Source: CAD feature listing. Evaluate the final solid. Frame: model axes, mm. Face numbers are marked on the shaded views. A direction names the side the tool comes from. Round coordinates to 2 decimals unless told otherwise and drop trailing zeros. Order: outer loops, then holes, each group sorted by start corner. A loop starts at its lowest first (then second) coordinate and runs counter-clockwise, first axis right, second up. Notation, with made-up numbers: (-21, 69) - (19, 69) arc R18 cw to (19, 75) - close; hole circle Ø9 at (-34, 44.5). An arc over 180 degrees is marked (long way). Use one line per item in the form item = value. Start each with the question number.
Q1. Cut plane A-A, the plane y = 36. Return the cut outline in (x, z), and give its area (3 significant figures).
Q2. Pin query (flat end, axial travel): pin 1 Ø12.5 at (x, z) = (56, 22) entering from +Y; pin 2 Ø16 at (y, z) = (42, 16) entering from +X; pin 3 Ø1 at (y, z) = (17.5, 43) entering from +X. Return the tip coordinate at first contact, or that it passes through.
Q3. Set-up query: the marked faces 1, 2 and 3. Return all of +Z, -Z, +X, -X, +Y, -Y with unobstructed straight access to the full face (end or side cutting, diameter ignored); none if empty.
Q4. Cut plane B-B, the plane z = 72.5. Return the cut outline in (x, y).
Q5. Ray query, line 1 (Y direction, x = 72.5, z = 74); line 2 (X direction, y = 39.5, z = 22.5); line 3 (Y direction, x = 43.5, z = 15). Return the intervals inside material, ascending. Write a range as [from, to].
Autodesk Inventor part; units mm, degrees
ref_plane "YZ Plane" through (0, 0, 0) normal (1, 0, 0) x (0, 1, 0)
ref_plane "XZ Plane" through (0, 0, 0) normal (0, 1, 0) x (-1, 0, 0)
ref_plane "XY Plane" through (0, 0, 0) normal (0, 0, 1) x (1, 0, 0)
sketch "스케치1" plane through (0, 0, 0) normal (0, 0, 1) x (1, 0, 0)
  line L0 (82.4719, -52.3014) -> (-82.4719, -52.3014)
  line L1 (-82.4719, -52.3014) -> (-82.4719, 52.3014)
  line L2 (-82.4719, 52.3014) -> (82.4719, 52.3014)
  line L3 (82.4719, 52.3014) -> (82.4719, -52.3014)
  line L4 (82.4719, -52.3014) -> (-82.4719, 52.3014) construction
  line L5 (-82.4719, -52.3014) -> (82.4719, 52.3014) construction
  point P0 (0, 0)
extrude "돌출1" add sketch "스케치1" along normal blind 100
sketch "스케치2" plane through (-82.4719, 52.3014, 0) normal (0, 1, 0) x (1, 0, 0)
  line L0 (164.9439, 0) -> (0, 0)
  line L1 (164.9439, 0) -> (116.2257, 0)
  line L2 (116.2257, 0) -> (116.2257, -42.2338)
  line L3 (116.2257, -42.2338) -> (164.9439, -42.2338)
  line L4 (164.9439, -42.2338) -> (164.9439, 0)
  point P0 (82.4719, 0)
extrude "돌출2" cut sketch "스케치2" against normal blind 20
sketch "스케치3" plane through (-82.4719, 52.3014, 100) normal (0, 1, 0) x (1, 0, 0)
  line L0 (164.9439, 0) -> (0, 0)
  line L1 (164.9439, 57.7662) -> (116.2257, 57.7662)
  line L2 (75.3221, 0) -> (164.9439, 0)
  line L3 (164.9439, 0) -> (164.9439, 57.7662)
  line L4 (164.9439, 57.7662) -> (75.3221, 57.7662)
  line L5 (75.3221, 57.7662) -> (75.3221, 0)
  point P0 (82.4719, 100)
extrude "돌출3" cut sketch "스케치3" against normal blind 50
properties part number "240503_3Dsketch03"
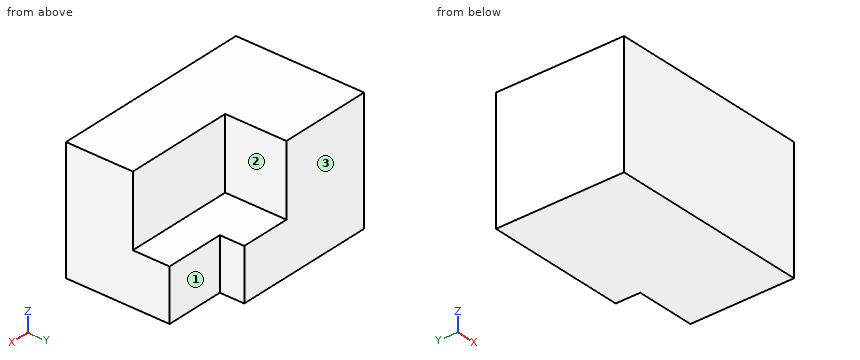
Completed:
q1.outline = (-82.47, 0) - (33.75, 0) - (33.75, 42.23) - (-7.15, 42.23) - (-7.15, 100) - (-82.47, 100) - close
q1.area = 9,260 mm2
q2.pin_1 = 32.3
q2.pin_2 = 33.75
q2.pin_3 = -7.15
q3.face_1 = +Z, -Z, +X, +Y
q3.face_2 = +Z, +X, +Y
q3.face_3 = +Z, -Z, +X, -X, +Y
q4.outline = (-82.47, -52.3) - (82.47, -52.3) - (82.47, 2.3) - (-7.15, 2.3) - (-7.15, 52.3) - (-82.47, 52.3) - close
q5.line_1 = [-52.3, 2.3]
q5.line_2 = [-82.47, 33.75]
q5.line_3 = [-52.3, 32.3]
